```python
from build123d import *

# Parameters (mm, degrees)
SKETCH1_R           = 50
BOSS_EXTRUDE1_DEPTH = 5
SKETCH2_R           = 9.5
SKETCH2_R_2         = 0.5
CUT_EXTRUDE1_DEPTH  = 5


with BuildPart() as part:
    # Sketch1 → Boss-Extrude1 (new body)
    with BuildSketch(Plane(origin=(0, 0, 0), x_dir=(1, 0, 0), z_dir=(0, 1, 0))):
        Circle(SKETCH1_R)
    extrude(amount=BOSS_EXTRUDE1_DEPTH)

    # Sketch2 → Cut-Extrude1 (cut)
    with BuildSketch(Plane(origin=(0, 5, 0), x_dir=(1, 0, 0), z_dir=(0, 1, 0))):
        with Locations((0, 32.614161607)):
            Circle(SKETCH2_R)
        Circle(SKETCH2_R_2)
        with Locations((23.061694835, 23.061694835)):
            Circle(SKETCH2_R)
        with Locations((32.614161607, 0)):
            Circle(SKETCH2_R)
        with Locations((23.061694835, -23.061694835)):
            Circle(SKETCH2_R)
        with Locations((0, -32.614161607)):
            Circle(SKETCH2_R)
        with Locations((-23.061694835, -23.061694835)):
            Circle(SKETCH2_R)
        with Locations((-32.614161607, 0)):
            Circle(SKETCH2_R)
        with Locations((-23.061694835, 23.061694835)):
            Circle(SKETCH2_R)
    extrude(amount=-CUT_EXTRUDE1_DEPTH, mode=Mode.SUBTRACT)


solid = part.part
```
Geometry check sheet. Reference: the model listing, model coordinates, mm. Give positions to 0.01 mm unless a question says otherwise; leave off trailing zeros. Write each loop counter-clockwise with the first axis right and the second up, starting at its lowest first coordinate (ties: lowest second). Pieces come first, ordered by that corner, then holes.
1) Gauge pin test, flat ends, axial feed: pin 1 (24.5 mm diameter, centred on x = 0, z = 32.61, fed in from -Y); pin 2 (1.5 mm diameter, centred on x = -28, y = 1, fed in from +Z). Record the tip position at first contact, or that the pin passes through.
2) Section check A-A, the plane x = -6.5. Record the boundary of the cut face in (y, z), and give its area (3 significant figures).
3) Section check B-B, the plane z = 37.5. Record the boundary of the cut face in (x, y).
4) Section check C-C, the plane y = 1.4. State how many separate pieces and enclosed holes the cut face has, and give its area (3 significant figures).
5) Material ranges on L1, parallel to Z at x = 0, y = 1.15; L2, parallel to X at y = 0.5, z = -21, recorded low to high.
6) Section check D-D, the plane x = 6. Record the boundary of the cut face in (y, z).
7) Release check for a two-part mould opening along X. For faces 1 (the cylindrical face through (47.69, 2.46, -15.02)), 2 (the flat face through (-1, 5, -1)), 3 (the cylindrical face through (-2.06, 2.54, -23.34)) record: pulls with the +X half, pulls with the -X half, needs draft (parallel to the pull), parting line crosses it, or undercut.
Computed:
1. pin 1: stops at y = 0
1. pin 2: stops at z = 41.92
2. outline: (0, -49.58) - (5, -49.58) - (5, -39.54) - (0, -39.54) - close; (0, -25.69) - (5, -25.69) - (5, 25.69) - (0, 25.69) - close; (0, 39.54) - (5, 39.54) - (5, 49.58) - (0, 49.58) - close
2. area: 357 mm2
3. outline: (-33.07, 0) - (-8.15, 0) - (-8.15, 5) - (-33.07, 5) - close; (8.15, 0) - (33.07, 0) - (33.07, 5) - (8.15, 5) - close
4. separate pieces: 1
4. enclosed holes: 9
4. area: 5,580 mm2
5. L1: z = -50 to -42.11, -23.11 to -0.5, 0.5 to 23.11, 42.11 to 50
5. L2: x = -45.38 to -32.34, -13.79 to 13.79, 32.34 to 45.38
6. outline: (0, -49.64) - (5, -49.64) - (5, -39.98) - (0, -39.98) - close; (0, -25.25) - (5, -25.25) - (5, 25.25) - (0, 25.25) - close; (0, 39.98) - (5, 39.98) - (5, 49.64) - (0, 49.64) - close
7. face 1: parting line crosses it
7. face 2: needs draft
7. face 3: undercut
